Read the model definition and answer for the solid it produces. Units are mm, in the model's axes. A direction names the side the tool comes from. Coordinates: 2 decimals unless noted, no trailing zeros. Order: outer loops, then holes, each group sorted by start corner. A loop starts at its lowest first (then second) coordinate and runs counter-clockwise, first axis right, second up. Notation, with made-up numbers: M 38.5,15.5 L 97.5,15.5 A10 cw 97.5,25.5 Z; hole C 35.5,56 d9. An arc over 180 degrees is marked long. One line per question, with ' | ' between items. Start each with the question number.
1) Find section A-A, the plane z = 71.5. Write down the section's boundary in (x, y).
2) A tool of negligible diameter and unlimited length cuts with its end or side. For faces 1 (the face through (-285.459, -139.688, 0.558)), 2 (the face through (-277.4, -1.07, 21.46)), 3 (the face through (-260.02, 131.47, 107.29)), from which of +Z, -Z, +X, -X, +Y, -Y can it reach the whole face along a straight path? Write none if from no direction.
3) Given P1, Ø6, axis at x = -214, y = 124.5, coming from the -Z side; P2, Ø4, axis at x = -130.5, z = 28.5, coming from the -Y side, each flat-ended and moving along its own axis, determine where each tip first touches the part or whether it passes through.
4) Consider probe 1 along Y at (x, z) = (205.5, -2); probe 2 along Y at (x, z) = (184.5, -15.5); probe 3 along Z at (x, y) = (-181, 140.5). Determine where each line is inside the solid, lowest interval first.
from build123d import *

# Parameters (mm, degrees)
F0_R     = 31.75
F3_R     = 12.7
F4_DEPTH = 304.8
F5_R     = 25.4
F6_DEPTH = 203.2


with BuildPart() as f2:
    # F2: sweep along a path in F1
    with BuildLine(Plane.XY) as f2_path:
        ThreePointArc((-203.2, 127), (-239.121024, 112.121024), (-254, 76.2))
        Line((-254, 76.2), (-254, -76.2))
        ThreePointArc((-254, -76.2), (-239.121024, -112.121024), (-203.2, -127))
        Line((-203.2, -127), (203.2, -127))
        ThreePointArc((203.2, -127), (239.121024, -112.121024), (254, -76.2))
        Line((254, -76.2), (254, 76.2))
        ThreePointArc((254, 76.2), (239.121024, 112.121024), (203.2, 127))
        Line((203.2, 127), (-203.2, 127))
    # F0 (on Front) → F2 (sweep)
    with BuildSketch(Plane.XZ):
        with Locations((-254, 0)):
            Circle(F0_R)
    sweep(path=f2_path.line)

    # F3 (on Right) → F4 (join)
    with BuildSketch(Plane.YZ):
        with Locations((-127, 0)):
            Circle(F3_R)
    extrude(amount=-F4_DEPTH)

    # F5 (on Top) → F6 (join)
    with BuildSketch(Plane.XY):
        with Locations((-241.3, 114.3)):
            Circle(F5_R)
    extrude(amount=F6_DEPTH)


solid = f2.part
Report:
1) outline: C -241.3,114.3 d50.8
2) face 1: -X | face 2: none | face 3: +Z
3) P1: stops at z = -31.75 | P2: stops at y = -144.49
4) probe 1: y = -158.65 to -95.17, 95.17 to 158.65 | probe 2: y = -154.71 to -99.29, 99.29 to 154.71 | probe 3: z = -28.74 to 28.74
